Source: CAD feature listing. Evaluate the final solid. Frame: model axes, mm. Face numbers are marked on the shaded views. Give positions to 0.01 mm unless a question says otherwise; leave off trailing zeros. Order: outer loops, then holes, each group sorted by start corner. A loop starts at its lowest first (then second) coordinate and runs counter-clockwise, first axis right, second up. Notation, with made-up numbers: M 37,55.5 L 93,55.5 A14 cw 93,63.5 Z; hole C 40.5,-21 d8. An arc over 180 degrees is marked long. Answer as a JSON object with one key per item and string values. Group by question number.
1. Section query B-B (z = 10.75). Output: boundary loops of the cut face in (x, y).
2. Section query C-C (y = -8.25). Output: boundary loops of the cut face in (x, z), plus the area to 3 significant figures.
3. Material intervals for L1, parallel to Y at x = 9, z = 18.5; L2, parallel to X at y = 3.5, z = 2.25; L3, parallel to X at y = 4, z = 8.5, sorted ascending. Write a range as [from, to].
4. Section query A-A (x = 11.25). Output: boundary loops of the cut face in (y, z).
5. Pin query (flat end, axial travel): P1, Ø1.5, axis at x = 16, y = 5.5, coming from the -Z side; P2, Ø8, axis at x = 1, y = -0.5, coming from the -Z side. Return the tip coordinate at first contact, or that it passes through.
6. Pull-direction query (Y, two-part tool) for the marked faces 1, 2 and 3; classes: +Y half, -Y half, draft (parallel to the pull), parting line (faces both ways), or undercut.
7. Section query D-D (y = 7.75). Output: boundary loops of the cut face in (x, z), plus the area to 3 significant figures.
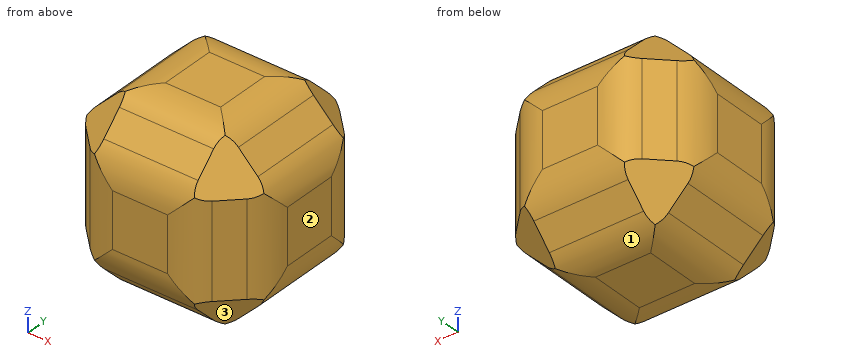
from build123d import *

# Parameters (mm, degrees)
F0_W        = 20
F0_H        = 20
F1_DEPTH    = 20
F2_SIZE     = 5
F3_T1_DEPTH = 20.3553390593
F3_T3_DEPTH = 20.3553390593
F3_T5_DEPTH = 20.3553390593


# Not quite as in the source:
# - a fillet or chamfer that OpenCascade refuses, or shapes differently, is made with other operations: its cross-section is extruded or revolved along the edge and cut away or added


with BuildPart() as f1:
    # F0 (on Top) → F1 (new body)
    with BuildSketch(Plane.XY):
        with Locations((8.6001078598, -0.1764608825)):
            Rectangle(F0_W, F0_H)
    extrude(amount=F1_DEPTH)

    # F2
    f2_edges = [f1.edges().sort_by_distance(p)[0] for p in [
        (8.600108, -10.176461, 20),
        (18.600108, -0.176461, 20),
        (8.600108, 9.823539, 20),
        (-1.399892, -0.176461, 20),
        (-1.399892, -0.176461, 0),
        (8.600108, 9.823539, 0),
        (18.600108, -0.176461, 0),
        (8.600108, -10.176461, 0),
        (-1.399892, 9.823539, 10),
        (18.600108, 9.823539, 10),
        (18.600108, -10.176461, 10),
        (-1.399892, -10.176461, 10),
    ]]
    chamfer(f2_edges, length=F2_SIZE)

    # F3: fillet of radius 5 on 24 edges, made by hand

    # F3_s2 → F3_t1 (cut)
    with BuildSketch(Plane.XZ.offset(-10.0012086472)):
        with BuildLine():
            ThreePointArc((11.529040048, 0), (13.4424572098, 0.3806023374), (15.0645739539, 1.4644660941))
            Line((15.0645739539, 1.4644660941), (13.6001078598, 0))
            Line((13.6001078598, 0), (11.529040048, 0))
        make_face()
        with BuildLine():
            ThreePointArc((18.6001078598, 7.0710678119), (18.2195055224, 5.15765065), (17.1356417658, 3.5355339059))
            Line((17.1356417658, 3.5355339059), (18.6001078598, 5))
            Line((18.6001078598, 5), (18.6001078598, 7.0710678119))
        make_face()
        with BuildLine():
            ThreePointArc((18.6001078598, 12.9289321881), (18.2195055224, 14.84234935), (17.1356417658, 16.4644660941))
            Line((17.1356417658, 16.4644660941), (18.6001078598, 15))
            Line((18.6001078598, 15), (18.6001078598, 12.9289321881))
        make_face()
        with BuildLine():
            ThreePointArc((11.529040048, 20), (13.4424572098, 19.6193976626), (15.0645739539, 18.5355339059))
            Line((15.0645739539, 18.5355339059), (13.6001078598, 20))
            Line((13.6001078598, 20), (11.529040048, 20))
        make_face()
        with BuildLine():
            ThreePointArc((5.6711756717, 20), (3.7577585099, 19.6193976626), (2.1356417658, 18.5355339059))
            Line((2.1356417658, 18.5355339059), (3.6001078598, 20))
            Line((3.6001078598, 20), (5.6711756717, 20))
        make_face()
        with BuildLine():
            ThreePointArc((-1.3998921402, 12.9289321881), (-1.0192898027, 14.84234935), (0.0645739539, 16.4644660941))
            Line((0.0645739539, 16.4644660941), (-1.3998921402, 15))
            Line((-1.3998921402, 15), (-1.3998921402, 12.9289321881))
        make_face()
        with BuildLine():
            ThreePointArc((-1.3998921402, 7.0710678119), (-1.0192898027, 5.15765065), (0.0645739539, 3.5355339059))
            Line((0.0645739539, 3.5355339059), (-1.3998921402, 5))
            Line((-1.3998921402, 5), (-1.3998921402, 7.0710678119))
        make_face()
        with BuildLine():
            ThreePointArc((5.6711756717, 0), (3.7577585099, 0.3806023374), (2.1356417658, 1.4644660941))
            Line((2.1356417658, 1.4644660941), (3.6001078598, 0))
            Line((3.6001078598, 0), (5.6711756717, 0))
        make_face()
    extrude(amount=F3_T1_DEPTH, mode=Mode.SUBTRACT)

    # F3_s4 → F3_t3 (cut)
    with BuildSketch(Plane.YZ.offset(-1.5775616698)):
        with BuildLine():
            ThreePointArc((9.8235391175, 7.0710678119), (9.4429367801, 5.15765065), (8.3590730234, 3.5355339059))
            Line((8.3590730234, 3.5355339059), (9.8235391175, 5))
            Line((9.8235391175, 5), (9.8235391175, 7.0710678119))
        make_face()
        with BuildLine():
            ThreePointArc((9.8235391175, 12.9289321881), (9.4429367801, 14.84234935), (8.3590730234, 16.4644660941))
            Line((8.3590730234, 16.4644660941), (9.8235391175, 15))
            Line((9.8235391175, 15), (9.8235391175, 12.9289321881))
        make_face()
        with BuildLine():
            ThreePointArc((6.2880052116, 1.4644660941), (4.6658884675, 0.3806023374), (2.7524713056, 0))
            Line((2.7524713056, 0), (4.8235391175, 0))
            Line((4.8235391175, 0), (6.2880052116, 1.4644660941))
        make_face()
        with BuildLine():
            ThreePointArc((-3.1053930706, 0), (-5.0188102325, 0.3806023374), (-6.6409269766, 1.4644660941))
            Line((-6.6409269766, 1.4644660941), (-5.1764608825, 0))
            Line((-5.1764608825, 0), (-3.1053930706, 0))
        make_face()
        with BuildLine():
            ThreePointArc((-8.7119947884, 3.5355339059), (-9.795858545, 5.15765065), (-10.1764608825, 7.0710678119))
            Line((-10.1764608825, 7.0710678119), (-10.1764608825, 5))
            Line((-10.1764608825, 5), (-8.7119947884, 3.5355339059))
        make_face()
        with BuildLine():
            ThreePointArc((-8.7119947884, 16.4644660941), (-9.795858545, 14.84234935), (-10.1764608825, 12.9289321881))
            Line((-10.1764608825, 12.9289321881), (-10.1764608825, 15))
            Line((-10.1764608825, 15), (-8.7119947884, 16.4644660941))
        make_face()
        with BuildLine():
            ThreePointArc((-3.1053930706, 20), (-5.0188102325, 19.6193976626), (-6.6409269766, 18.5355339059))
            Line((-6.6409269766, 18.5355339059), (-5.1764608825, 20))
            Line((-5.1764608825, 20), (-3.1053930706, 20))
        make_face()
        with BuildLine():
            ThreePointArc((6.2880052116, 18.5355339059), (4.6658884675, 19.6193976626), (2.7524713056, 20))
            Line((2.7524713056, 20), (4.8235391175, 20))
            Line((4.8235391175, 20), (6.2880052116, 18.5355339059))
        make_face()
    extrude(amount=F3_T3_DEPTH, mode=Mode.SUBTRACT)

    # F3_s6 → F3_t5 (cut)
    with BuildSketch(Plane.XY.offset(-0.1776695297)):
        with BuildLine():
            ThreePointArc((0.0645739539, 6.2880052116), (-1.0192898027, 4.6658884675), (-1.3998921402, 2.7524713056))
            Line((-1.3998921402, 2.7524713056), (-1.3998921402, 4.8235391175))
            Line((-1.3998921402, 4.8235391175), (0.0645739539, 6.2880052116))
        make_face()
        with BuildLine():
            ThreePointArc((5.6711756717, 9.8235391175), (3.7577585099, 9.4429367801), (2.1356417658, 8.3590730234))
            Line((2.1356417658, 8.3590730234), (3.6001078598, 9.8235391175))
            Line((3.6001078598, 9.8235391175), (5.6711756717, 9.8235391175))
        make_face()
        with BuildLine():
            ThreePointArc((11.529040048, 9.8235391175), (13.4424572098, 9.4429367801), (15.0645739539, 8.3590730234))
            Line((15.0645739539, 8.3590730234), (13.6001078598, 9.8235391175))
            Line((13.6001078598, 9.8235391175), (11.529040048, 9.8235391175))
        make_face()
        with BuildLine():
            ThreePointArc((17.1356417658, 6.2880052116), (18.2195055224, 4.6658884675), (18.6001078598, 2.7524713056))
            Line((18.6001078598, 2.7524713056), (18.6001078598, 4.8235391175))
            Line((18.6001078598, 4.8235391175), (17.1356417658, 6.2880052116))
        make_face()
        with BuildLine():
            ThreePointArc((18.6001078598, -3.1053930706), (18.2195055224, -5.0188102325), (17.1356417658, -6.6409269766))
            Line((17.1356417658, -6.6409269766), (18.6001078598, -5.1764608825))
            Line((18.6001078598, -5.1764608825), (18.6001078598, -3.1053930706))
        make_face()
        with BuildLine():
            ThreePointArc((15.0645739539, -8.7119947884), (13.4424572098, -9.795858545), (11.529040048, -10.1764608825))
            Line((11.529040048, -10.1764608825), (13.6001078598, -10.1764608825))
            Line((13.6001078598, -10.1764608825), (15.0645739539, -8.7119947884))
        make_face()
        with BuildLine():
            ThreePointArc((2.1356417658, -8.7119947884), (3.7577585099, -9.795858545), (5.6711756717, -10.1764608825))
            Line((5.6711756717, -10.1764608825), (3.6001078598, -10.1764608825))
            Line((3.6001078598, -10.1764608825), (2.1356417658, -8.7119947884))
        make_face()
        with BuildLine():
            ThreePointArc((-1.3998921402, -3.1053930706), (-1.0192898027, -5.0188102325), (0.0645739539, -6.6409269766))
            Line((0.0645739539, -6.6409269766), (-1.3998921402, -5.1764608825))
            Line((-1.3998921402, -5.1764608825), (-1.3998921402, -3.1053930706))
        make_face()
    extrude(amount=F3_T5_DEPTH, mode=Mode.SUBTRACT)


solid = f1.part
Answer sheet:
{
 "1": {"outline": "M -1.4,-3.11 A5 ccw 0.06,-6.64 L 2.14,-8.71 A5 ccw 5.67,-10.18 L 11.53,-10.18 A5 ccw 15.06,-8.71 L 17.14,-6.64 A5 ccw 18.6,-3.11 L 18.6,2.75 A5 ccw 17.14,6.29 L 15.06,8.36 A5 ccw 11.53,9.82 L 5.67,9.82 A5 ccw 2.14,8.36 L 0.06,6.29 A5 ccw -1.4,2.75 Z"},
 "2": {"outline": "M 1.67,5 L 3.6,3.07 L 13.6,3.07 L 15.53,5 L 15.53,15 L 13.6,16.93 L 3.6,16.93 L 1.67,15 Z", "area": "184 mm^2"},
 "3": {"L1": "[-6.68, 6.32]", "L2": "[1.35, 15.85]", "L3": "[-1.24, 18.44]"},
 "4": {"outline": "M -10.18,7.07 A5 ccw -8.71,3.54 L -6.64,1.46 A5 ccw -3.11,0 L 2.75,0 A5 ccw 6.29,1.46 L 8.36,3.54 A5 ccw 9.82,7.07 L 9.82,12.93 A5 ccw 8.36,16.46 L 6.29,18.54 A5 ccw 2.75,20 L -3.11,20 A5 ccw -6.64,18.54 L -8.71,16.46 A5 ccw -10.18,12.93 Z"},
 "5": {"P1": "z = 2.02", "P2": "z = 0.05"},
 "6": {"face 1": "+Y half", "face 2": "draft", "face 3": "-Y half"},
 "7": {"outline": "M 1.53,5 L 3.6,2.93 L 13.6,2.93 L 15.67,5 L 15.67,15 L 13.6,17.07 L 3.6,17.07 L 1.53,15 Z", "area": "192 mm^2"}
}
